Part model, mm, in its own coordinate system. A direction names the side the tool comes from. Give positions to 0.01 mm unless a question says otherwise; leave off trailing zeros. Write each loop counter-clockwise with the first axis right and the second up, starting at its lowest first coordinate (ties: lowest second). Pieces come first, ordered by that corner, then holes. Notation, with made-up numbers: (0.5, 79.25) - (28.5, 79.25) arc R7 ccw to (28.5, 87.25) - close; hole circle Ø2 at (18.25, 54.5). An arc over 180 degrees is marked (long way). Answer as a JSON object with one key per item and string values. Group by question number.
```python
from build123d import *

# Parameters (mm, degrees)
F0_W     = 90.20937762
F0_H     = 55.82251726
F1_DEPTH = 76.2
F2_R     = 16.9269763234
F3_DEPTH = 76.2
F4_W     = 51.9804880023
F4_H     = 10.2611703347
F5_DEPTH = 50.8
F6_R     = 7.62
F7_DEPTH = 50.8
F8_W     = 9.5572224044
F8_H     = 27.9414801582
F8_H_2   = 27.91125863
F9_DEPTH = 50.8
F10_R    = 1.27


with BuildPart() as f1:
    # F0 (on Top) → F1 (new body)
    with BuildSketch(Plane.XY):
        Rectangle(F0_W, F0_H)
    extrude(amount=F1_DEPTH)

    # F2 (on face) → F3 (cut)
    with BuildSketch(Plane.XY.offset(76.2)):
        with Locations((0, 27.91125863)):
            Circle(F2_R)
    extrude(amount=-F3_DEPTH, mode=Mode.SUBTRACT)

    # F4 (on face) → F5 (cut)
    with BuildSketch(Plane.XY.offset(76.2)):
        with Locations((0, -22.7806734627)):
            Rectangle(F4_W, F4_H)
    extrude(amount=-F5_DEPTH, mode=Mode.SUBTRACT)

    # F6 (on face) → F7 (cut)
    with BuildSketch(Plane.XY.offset(76.2)):
        with Locations((-29.86468881, 7.64874137)):
            Circle(F6_R)
        with Locations((29.86468881, 7.64874137)):
            Circle(F6_R)
    extrude(amount=-F7_DEPTH, mode=Mode.SUBTRACT)

    # F8 (on face) → F9 (cut)
    with BuildSketch(Plane.XY.offset(76.2)):
        with BuildLine():
            Line((-22.2841894419, 27.91125863), (-45.10468881, 27.91125863))
            Line((-45.10468881, 27.91125863), (-45.10468881, 6.8738676186))
            Line((-45.10468881, 6.8738676186), (-37.4451881781, 6.8738676186))
            ThreePointArc((-37.4451881781, 6.8738676186), (-30.6395625614, 15.2292407381), (-22.2841894419, 8.4236151214))
            Line((-22.2841894419, 8.4236151214), (-22.2841894419, 27.91125863))
        make_face()
        with BuildLine():
            Line((-37.4451881781, 6.8738676186), (-45.10468881, 6.8738676186))
            Line((-45.10468881, 6.8738676186), (-45.10468881, 0.0302215282))
            Line((-45.10468881, 0.0302215282), (-35.5474664056, 0.0302215282))
            Line((-35.5474664056, 0.0302215282), (-30.0148734284, 0.0302215282))
            ThreePointArc((-30.0148734284, 0.0302215282), (-35.0270275898, 2.0438632873), (-37.4451881781, 6.8738676186))
        make_face()
        with Locations((-40.3260776078, -13.9405185509)):
            Rectangle(F8_W, F8_H)
        with BuildLine():
            Line((45.10468881, 27.91125863), (22.2841894419, 27.91125863))
            Line((22.2841894419, 27.91125863), (22.2841894419, 8.4236151214))
            ThreePointArc((22.2841894419, 8.4236151214), (30.2526287637, 15.2588598048), (37.48468881, 7.64874137))
            ThreePointArc((37.48468881, 7.64874137), (37.4748072448, 7.2608014163), (37.4451881781, 6.8738676186))
            Line((37.4451881781, 6.8738676186), (45.10468881, 6.8738676186))
            Line((45.10468881, 6.8738676186), (45.10468881, 27.91125863))
        make_face()
        with BuildLine():
            Line((45.10468881, 0), (45.10468881, 6.8738676186))
            Line((45.10468881, 6.8738676186), (37.4451881781, 6.8738676186))
            ThreePointArc((37.4451881781, 6.8738676186), (34.9251180007, 1.9516845504), (29.7400578856, 0.0297606552))
            Line((29.7400578856, 0.0297606552), (29.7400578856, 0))
            Line((29.7400578856, 0), (35.5474664056, 0))
            Line((35.5474664056, 0), (45.10468881, 0))
        make_face()
        with Locations((40.3260776078, -13.955629315)):
            Rectangle(F8_W, F8_H_2)
    extrude(amount=-F9_DEPTH, mode=Mode.SUBTRACT)

    # F10
    f10_edges = [f1.edges().sort_by_distance(p)[0] for p in [
        (-33.694439, 27.911259, 25.4),
        (33.694439, 27.911259, 25.4),
        (19.605583, 27.911259, 76.2),
        (-19.605583, 27.911259, 76.2),
        (0, 10.984282, 76.2),
        (25.990244, -22.780673, 76.2),
        (30.768855, -27.911259, 76.2),
        (35.547466, -13.955629, 76.2),
        (32.643762, 0, 76.2),
        (29.740058, 0.01488, 76.2),
        (24.167632, 2.588312, 76.2),
        (22.284189, 18.167437, 76.2),
        (-22.284189, 18.167437, 76.2),
        (-24.259811, 2.486403, 76.2),
        (-32.78117, 0.030222, 76.2),
        (-35.547466, -13.940519, 76.2),
        (-30.768855, -27.911259, 76.2),
        (-25.990244, -22.780673, 76.2),
        (0, -17.650088, 76.2),
        (0, -27.911259, 25.4),
        (-40.326078, -27.911259, 25.4),
        (-45.104689, 0, 25.4),
        (45.104689, 0, 25.4),
        (40.326078, -27.911259, 25.4),
    ]]
    fillet(f10_edges, radius=F10_R)


solid = f1.part
```
1) Drill centre lines: line 1 along X through (y, z) = (-23, 37.5); line 2 along Z through (x, y) = (38, -5); line 3 along X through (y, z) = (-12, 41.5). Where is each one in solid material? Low to high. Write a range as from..to.
2) Saw through at C-C (z = 20). List the corners of the cut face in (x, y).
3) Saw through at B-B (y = -3.5). List the corners of the cut face in (x, z).
4) Two-plate mould, pull along X, no slides. Class faces 1 (the flat face through (-45.105, 0, 12)), 2 (the cylindrical face through (-0.37, 10.99, 37.99)), 3 (the flat face through (-33, 0.03, 51)): +X half, -X half, draft (parallel to the pull), parting line (faces both ways), or undercut.
5) Saw through at D-D (x = 19.5). List the corners of the cut face in (y, z).
6) Saw through at A-A (x = 0). List the corners of the cut face in (y, z).
7) Which spindle directions (+Z, -Z, +X, -X, +Y, -Y) get a long thin tool onto all of the face, cutting with end or side? Do faces 4 (the flat face through (22.284, 18, 50)), 5 (the flat face through (0, -17.65, 51)), 6 (the flat face through (-22.284, 18, 50)). Say none if no direction does.
8) Drop flat-ended pins along their axis: P1, Ø6, axis at x = 25, y = 19, coming from the +Z side; P2, Ø6, axis at x = -2, y = -14.5, coming from the -Z side; P3, Ø22.5, axis at y = -8.5, z = 56, coming from the -X side; P4, Ø8, axis at y = -21.5, z = 42.5, coming from the +X side. Give the stop position or say it passes through.
Checks:
{
 "1": {"line 1": "-35.55..-25.99, 25.99..35.55", "line 2": "0..25.4", "line 3": "-35.55..35.55"},
 "2": {"outline": "(-45.1, -27.91) - (45.1, -27.91) - (45.1, 27.91) - (16.93, 27.91) arc R16.93 cw to (-16.93, 27.91) - (-45.1, 27.91) - close"},
 "3": {"outline": "(-45.1, 0) - (45.1, 0) - (45.1, 24.13) arc R1.27 ccw to (43.83, 25.4) - (35.55, 25.4) - (35.55, 74.93) arc R1.27 ccw to (34.28, 76.2) - (-34.28, 76.2) arc R1.27 ccw to (-35.55, 74.93) - (-35.55, 25.4) - (-43.83, 25.4) arc R1.27 ccw to (-45.1, 24.13) - close"},
 "4": {"face 1": "-X half", "face 2": "undercut", "face 3": "draft"},
 "5": {"outline": "(-27.91, 0) - (27.91, 0) - (27.91, 74.93) arc R1.27 ccw to (26.64, 76.2) - (-16.38, 76.2) arc R1.27 ccw to (-17.65, 74.93) - (-17.65, 25.4) - (-26.64, 25.4) arc R1.27 ccw to (-27.91, 24.13) - close"},
 "6": {"outline": "(-27.91, 0) - (10.98, 0) - (10.98, 74.93) arc R1.27 ccw to (9.71, 76.2) - (-16.38, 76.2) arc R1.27 ccw to (-17.65, 74.93) - (-17.65, 25.4) - (-26.64, 25.4) arc R1.27 ccw to (-27.91, 24.13) - close"},
 "7": {"face 4": "+Z, +X, +Y", "face 5": "+Z, -Y", "face 6": "+Z, -X, +Y"},
 "8": {"P1": "z = 75.73", "P2": "z = 0", "P3": "x = -35.55", "P4": "x = 35.55"}
}
